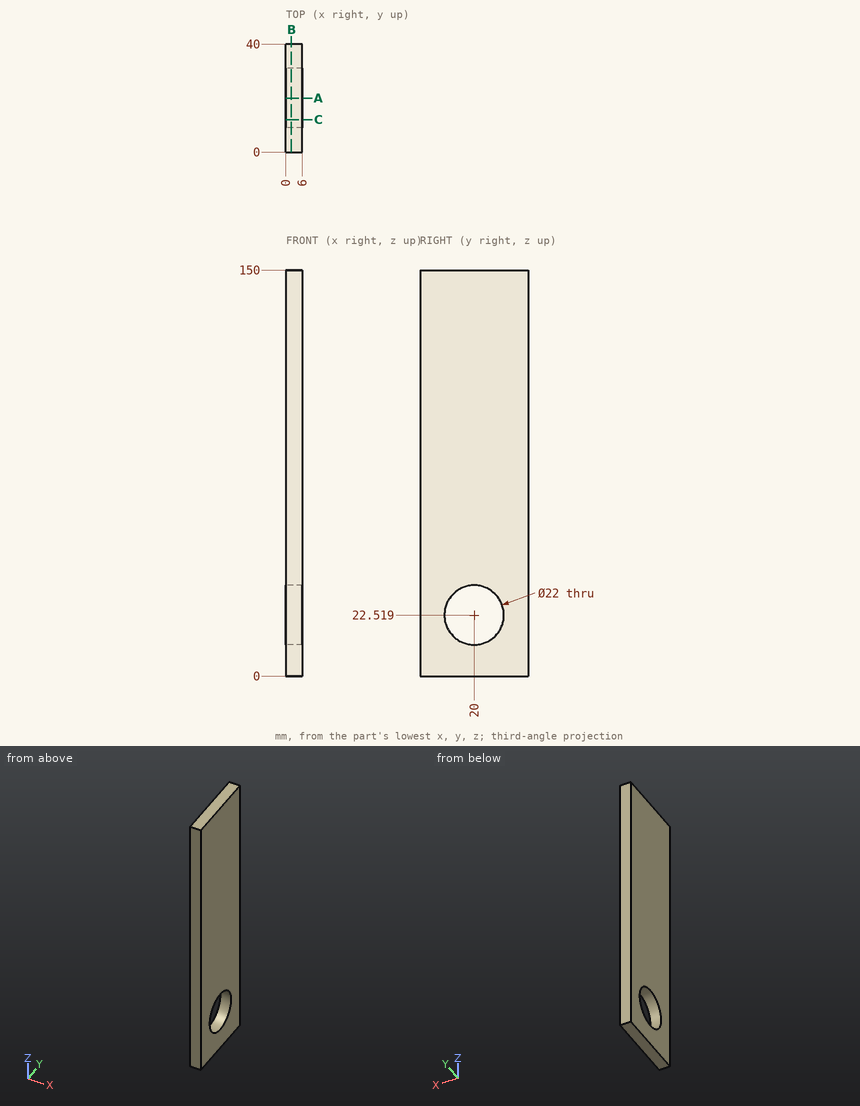
Study the drawing (mm; zero at the part's minimum x, y, z) and answer. Give positions to 0.01 mm unless a question says otherwise; leave off trailing zeros. Write each loop counter-clockwise with the first axis right and the second up, starting at its lowest first coordinate (ties: lowest second). Pieces come first, ordered by that corner, then holes. Notation, with made-up numbers: (23, 3) - (38, 3) arc R10 cw to (38, 11) - close; hole circle Ø1 at (80.5, 13.25). An arc over 180 degrees is marked (long way). Use a Markdown table: item, result.
1. Section B-B on x = 2.1 is taken. Write down the section's boundary in (y, z).
Values follow:
| item | result |
|---|---|
| outline | (0, 0) - (40, 0) - (40, 150) - (0, 150) - close; hole circle Ø22 at (20, 22.52) |
2. Find the intervals of material crossed by probe 1 along Z at (x, y) = (4.8, 20.5); probe 2 along Y at (x, z) = (1.75, 22); probe 3 along Y at (x, z) = (3.45, 24.5), in increasing order. Write a range as from..to.
Values follow:
| item | result |
|---|---|
| probe 1 | z = 0..11.53, 33.51..150 |
| probe 2 | y = 0..9.01, 30.99..40 |
| probe 3 | y = 0..9.18, 30.82..40 |
3. Section A-A on y = 20 is taken. Write down the section's boundary in (x, z), plus the area to 3 significant figures.
Values follow:
| item | result |
|---|---|
| outline | (0, 0) - (6, 0) - (6, 11.52) - (0, 11.52) - close; (0, 33.52) - (6, 33.52) - (6, 150) - (0, 150) - close |
| area | 768 mm² |
4. Section C-C on y = 12 is taken. Write down the section's boundary in (x, z).
Values follow:
| item | result |
|---|---|
| outline | (0, 0) - (6, 0) - (6, 14.97) - (0, 14.97) - close; (0, 30.07) - (6, 30.07) - (6, 150) - (0, 150) - close |
